The listing builds one solid part. Answer for the finished solid, in the listing's coordinates (mm). Give positions to 0.01 mm unless a question says otherwise; leave off trailing zeros. Order: outer loops, then holes, each group sorted by start corner. A loop starts at its lowest first (then second) coordinate and runs counter-clockwise, first axis right, second up. Notation, with made-up numbers: (2.25, -7) - (61.25, -7) arc R8 cw to (61.25, -1) - close; hole circle Ø7 at (32, 84.5). An arc over 180 degrees is marked (long way). Answer in a Markdown table with one row per item. Add a question column.
Autodesk Inventor part; units mm, degrees
ref_plane "YZ Plane" through (0, 0, 0) normal (1, 0, 0) x (0, 1, 0)
ref_plane "XZ Plane" through (0, 0, 0) normal (0, 1, 0) x (-1, 0, 0)
ref_plane "XY Plane" through (0, 0, 0) normal (0, 0, 1) x (1, 0, 0)
sketch "Sketch1" plane through (0, 0, 0) normal (0, 0, 1) x (1, 0, 0)
  line L0 (0, 0) -> (0, 400)
  line L1 (0, 400) -> (4, 400)
  line L2 (4, 400) -> (4, 385)
  line L3 (4, 385) -> (5, 385)
  line L4 (5, 385) -> (5, 346)
  line L5 (5, 346) -> (6, 346)
  line L6 (6, 346) -> (6, 10)
  line L7 (6, 10) -> (4, 10)
  line L8 (4, 10) -> (4, 0)
  line L9 (4, 0) -> (0, 0)
  dimension "d0" = 400
  dimension "d1" = 8
  dimension "d2" = 10
  dimension "d3" = 12
  dimension "d4" = 10
  dimension "d5" = 8
  dimension "d6" = 15
  dimension "d7" = 39
revolve "Revolution1" add sketch "Sketch1" angle 360 about axis through (0, 0, 0) along (0, 1, 0)
thread "Thread1"
properties part number "Z Axis Ball Screw" material "Stainless Steel"
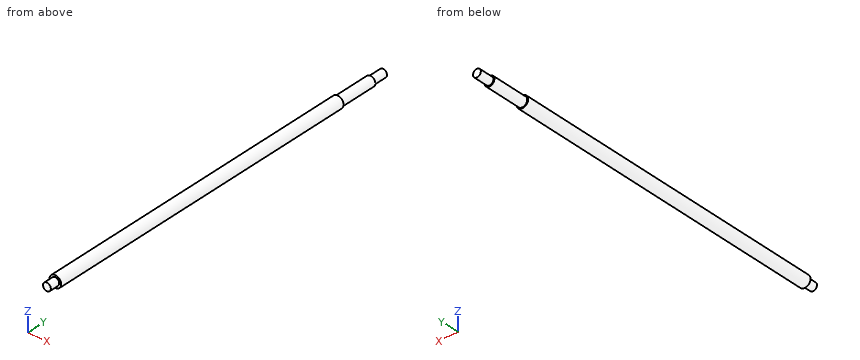
(1) Find section C-C, the plane y = 231. Write down the section's boundary in (x, z).
(2) Find section A-A, the plane z = 0. Write down the section's boundary in (x, y), plus the area to 3 significant figures.
(3) Find section B-B, the plane x = 0. Write down the section's boundary in (y, z), plus the area to 3 significant figures.
(4) Straight lines are drawn through the part: line 1 (Y direction, x = -4.25, z = 2.75); line 2 (Y direction, x = -0.5, z = 4); line 3 (X direction, y = 235, z = 0.75). For each, find the intervals that lie inside material, in ascending order.
(5) Each of these flat-tipped pins is pushed along its axis until it touches: P1, Ø6, axis at x = -3.5, z = -2, coming from the -Y side; P2, Ø6, axis at y = 236, z = -4.5, coming from the -X side; P3, Ø3, axis at y = 272, z = -4, coming from the -X side; P4, Ø5, axis at y = 352.5, z = 4.5, coming from the -X side. Where does it stop, or does it pass through?
Answer key:
| question | item | result |
|---|---|---|
| 1 | outline | circle Ø12 at (0, 0) |
| 2 | outline | (-6, 10) - (-4, 10) - (-4, 0) - (4, 0) - (4, 10) - (6, 10) - (6, 346) - (5, 346) - (5, 385) - (4, 385) - (4, 400) - (-4, 400) - (-4, 385) - (-5, 385) - (-5, 346) - (-6, 346) - close |
| 2 | area | 4,620 mm² |
| 3 | outline | (0, -4) - (10, -4) - (10, -6) - (346, -6) - (346, -5) - (385, -5) - (385, -4) - (400, -4) - (400, 4) - (385, 4) - (385, 5) - (346, 5) - (346, 6) - (10, 6) - (10, 4) - (0, 4) - close |
| 3 | area | 4,620 mm² |
| 4 | line 1 | 10 to 346 |
| 4 | line 2 | 10 to 385 |
| 4 | line 3 | -5.95 to 5.95 |
| 5 | P1 | y = 0 |
| 5 | P2 | x = -5.81 |
| 5 | P3 | x = -5.45 |
| 5 | P4 | x = -4.58 |
